from build123d import *

# Parameters (mm, degrees)
F0_W     = 66.04
F0_H     = 62.23
F1_DEPTH = 4.7625
F2_R     = 2.0828
F2_W     = 23.6109700747
F2_H     = 10.16
F2_W_2   = 21.1328
F3_DEPTH = 25.4


with BuildPart() as f1:
    # F0 (on Top) → F1 (new body)
    with BuildSketch(Plane.XY):
        Rectangle(F0_W, F0_H)
    extrude(amount=F1_DEPTH)

    # F2 (on face) → F3 (cut)
    with BuildSketch(Plane.XY.offset(4.7625)):
        with Locations((-26.4963417654, 26.4567458333)):
            Circle(F2_R)
        with BuildLine():
            ThreePointArc((18.1444912354, 26.4567458333), (16.0616912354, 28.5395458333), (13.9788912354, 26.4567458333))
            ThreePointArc((13.9788912354, 26.4567458333), (16.0616912354, 24.3739458333), (18.1444912354, 26.4567458333))
        make_face()
        with BuildLine():
            ThreePointArc((24.0372912354, -0.2640541667), (23.4272532393, 1.2087078372), (21.9544912354, 1.8187458333))
            Line((21.9544912354, 1.8187458333), (21.9544912354, -2.3468541667))
            ThreePointArc((21.9544912354, -2.3468541667), (23.4272532393, -1.7368161705), (24.0372912354, -0.2640541667))
        make_face()
        with BuildLine():
            Line((21.9544912354, -2.3468541667), (21.9544912354, 1.8187458333))
            ThreePointArc((21.9544912354, 1.8187458333), (19.8716912354, -0.2640541667), (21.9544912354, -2.3468541667))
        make_face()
        with BuildLine():
            ThreePointArc((-20.7683087646, -0.2640541667), (-21.3783467607, 1.2087078372), (-22.8511087646, 1.8187458333))
            Line((-22.8511087646, 1.8187458333), (-22.8511087646, -2.3468541667))
            ThreePointArc((-22.8511087646, -2.3468541667), (-21.3783467607, -1.7368161705), (-20.7683087646, -0.2640541667))
        make_face()
        with BuildLine():
            Line((-22.8511087646, -2.3468541667), (-22.8511087646, 1.8187458333))
            ThreePointArc((-22.8511087646, 1.8187458333), (-24.9339087646, -0.2640541667), (-22.8511087646, -2.3468541667))
        make_face()
        with BuildLine():
            Line((-22.8511087646, -24.3432541667), (-22.8511087646, -28.5088541667))
            ThreePointArc((-22.8511087646, -28.5088541667), (-21.3783467607, -27.8988161705), (-20.7683087646, -26.4260541667))
            ThreePointArc((-20.7683087646, -26.4260541667), (-21.3783467607, -24.9532921628), (-22.8511087646, -24.3432541667))
        make_face()
        with BuildLine():
            ThreePointArc((-22.8511087646, -24.3432541667), (-24.9339087646, -26.4260541667), (-22.8511087646, -28.5088541667))
            Line((-22.8511087646, -28.5088541667), (-22.8511087646, -24.3432541667))
        make_face()
        with BuildLine():
            Line((21.9544912354, -24.3432541667), (21.9544912354, -28.5088541667))
            ThreePointArc((21.9544912354, -28.5088541667), (23.4272532393, -27.8988161705), (24.0372912354, -26.4260541667))
            ThreePointArc((24.0372912354, -26.4260541667), (23.4272532393, -24.9532921628), (21.9544912354, -24.3432541667))
        make_face()
        with BuildLine():
            ThreePointArc((21.9544912354, -24.3432541667), (19.8716912354, -26.4260541667), (21.9544912354, -28.5088541667))
            Line((21.9544912354, -28.5088541667), (21.9544912354, -24.3432541667))
        make_face()
        with Locations((-10.9837938019, 13.2487458333)):
            Rectangle(F2_W, F2_H)
        with Locations((11.3880912354, 13.2487458333)):
            Rectangle(F2_W_2, F2_H)
    extrude(amount=-F3_DEPTH, mode=Mode.SUBTRACT)


solid = f1.part
For this review, take the finished solid that the model builds, in its own axes (mm). A direction names the side the tool comes from. Give positions to 0.01 mm unless a question says otherwise; leave off trailing zeros. Order: outer loops, then holes, each group sorted by start corner. A loop starts at its lowest first (then second) coordinate and runs counter-clockwise, first axis right, second up. Notation, with made-up numbers: M 12,35 L 19,35 A36 ccw 19,73 Z; hole C 67.5,68.5 d11. An arc over 180 degrees is marked long. Answer in a Markdown table with one row per item. Add a question column.
(1) Consider section B-B on y = 17. State the section outline as (x, z) points.
(2) Consider section C-C on z = 2.5. State the section outline as (x, y) points (1 decimal).
(3) Consider section D-D on y = 1. State the section outline as (x, z) points.
(4) Wall thickness on probe 1 along X at (y, z) = (0, 1.3); probe 2 along Y at (x, z) = (10, 0.45) (3 decimals); probe 3 along X at (y, z) = (11.5, 0.7): over which ranges is each line inside the solid? List them lowest first. Write a range as [from, to].
(5) Consider section A-A on x = -9. State the section outline as (y, z) points (1 decimal).
(6) For faces 5 (the face through (0, -31.115, 2)), 6 (the face through (-1, 8.169, 2)), list the 3-axis set-ups (+Z, -Z, +X, -X, +Y, -Y) from which the entire face can be reached by the end or side of a thin tool; tool diameter is ignored.
(7) Mouldability with a two-part tool opening along Y and no side actions: class faces 1 (the face through (0, 31.115, 2)), 2 (the face through (0, 18.329, 2)), 3 (the face through (0, 0, 4.762)), 4 (the face through (-22.789, 13, 2)) as +Y half, -Y half, draft (parallel to the pull), parting line (faces both ways), or undercut.
Evaluation:
| question | item | result |
|---|---|---|
| 1 | outline | M -33.02,0 L -22.79,0 L -22.79,4.76 L -33.02,4.76 Z; M 21.95,0 L 33.02,0 L 33.02,4.76 L 21.95,4.76 Z |
| 2 | outline | M -33,-31.1 L 33,-31.1 L 33,31.1 L -33,31.1 Z; hole C -26.5,26.5 d4.2; hole C -22.9,-26.4 d4.2; hole C -22.9,-0.3 d4.2; hole M -22.8,8.2 L 22,8.2 L 22,18.3 L -22.8,18.3 Z; hole C 16.1,26.5 d4.2; hole C 22,-26.4 d4.2; hole C 22,-0.3 d4.2 |
| 3 | outline | M -33.02,0 L -24.51,0 L -24.51,4.76 L -33.02,4.76 Z; M -21.2,0 L 20.3,0 L 20.3,4.76 L -21.2,4.76 Z; M 23.61,0 L 33.02,0 L 33.02,4.76 L 23.61,4.76 Z |
| 4 | probe 1 | x = [-33.02, -24.92], [-20.79, 19.89], [24.02, 33.02] |
| 4 | probe 2 | y = [-31.115, 8.169], [18.329, 31.115] |
| 4 | probe 3 | x = [-33.02, -22.79], [21.95, 33.02] |
| 5 | outline | M -31.1,0 L 8.2,0 L 8.2,4.8 L -31.1,4.8 Z; M 18.3,0 L 31.1,0 L 31.1,4.8 L 18.3,4.8 Z |
| 6 | face 5 | +Z, -Z, +X, -X, -Y |
| 6 | face 6 | +Z, -Z |
| 7 | face 1 | +Y half |
| 7 | face 2 | undercut |
| 7 | face 3 | draft |
| 7 | face 4 | undercut |
